Could you check a few things on this model? Use its own coordinates, in mm. Give positions to 0.01 mm unless a question says otherwise; leave off trailing zeros. Loops run counter-clockwise (first coordinate to the right, second up) from the corner with the lowest first, then second, coordinate; pieces in that order, holes last. Notation, with made-up numbers: M 47.5,35.25 L 61.5,35.25 A29 cw 61.5,65.25 Z; hole C -15.5,75 d10. An arc over 180 degrees is marked long. Return JSON: item names as keys, results as strings. Group by question number.
1. If we section it at C-C (y = 14.5): Write out the boundary of the cut face in (x, z), plus the area to 3 significant figures.
2. If we section it at A-A (x = 45.5): Write out the boundary of the cut face in (y, z).
3. Please list where these lines run through material, in increasing order: line 1 (Y direction, x = 45.5, z = 1.3); line 2 (Y direction, x = 45, z = 1.2); line 3 (X direction, y = 27.5, z = 0.7).
4. For pin 1 (2.5 mm diameter, centred on x = 14.5, y = 14.5, fed in from -Z); pin 2 (5 mm diameter, centred on x = 45.5, y = 14.5, fed in from -Z), each with a flat end and sliding along its axis, tell me the tip position at first contact or that it passes through.
5. If we section it at D-D (y = 26.5): Write out the boundary of the cut face in (x, z), plus the area to 3 significant figures.
6. If we section it at B-B (z = 1.4): Write out the boundary of the cut face in (x, y).
```python
from build123d import *

# Parameters (mm, degrees)
CROQUIS1_W              = 60
CROQUIS1_H              = 60
SALIENTE_EXTRUIR1_DEPTH = 2
CROQUIS7_R              = 1.6
CORTAR_EXTRUIR1_DEPTH   = 85.876380696
CROQUIS8_OUTSIDE_W      = 78.976
CROQUIS8_OUTSIDE_H      = 78.976
CORTAR_EXTRUIR2_DEPTH   = 10
CORTAR_EXTRUIR4_DEPTH   = 73.859453745
CHAFL_N1_SIZE           = 4


with BuildPart() as part:
    # Croquis1 → Saliente-Extruir1 (new body)
    with BuildSketch(Plane.XY):
        with Locations((30, 30)):
            Rectangle(CROQUIS1_W, CROQUIS1_H)
    extrude(amount=SALIENTE_EXTRUIR1_DEPTH)

    # Croquis7 → Cortar-Extruir1 (cut, through all)
    with BuildSketch(Plane.XY.offset(2)):
        with Locations((14.5, 45.5)):
            Circle(CROQUIS7_R)
        with Locations((45.5, 45.5)):
            Circle(CROQUIS7_R)
        with Locations((14.5, 14.5)):
            Circle(CROQUIS7_R)
        with Locations((45.5, 14.5)):
            Circle(CROQUIS7_R)
    extrude(amount=-CORTAR_EXTRUIR1_DEPTH, mode=Mode.SUBTRACT)

    # Croquis8 outside → Cortar-Extruir2 (cut)
    with BuildSketch(Plane(origin=(0, 0, 0), x_dir=(-1, 0, 0), z_dir=(0, 0, -1))):
        with Locations((-30, 30)):
            Rectangle(CROQUIS8_OUTSIDE_W, CROQUIS8_OUTSIDE_H)
        with BuildLine():
            Line((-51.5, 51.5), (-51.5, 8.5))
            Line((-51.5, 8.5), (-8.5, 8.5))
            Line((-8.5, 8.5), (-8.5, 36.95))
            ThreePointArc((-8.5, 36.95), (-16.379748932, 42.703353122), (-20.6, 51.5))
            Line((-20.6, 51.5), (-51.5, 51.5))
        make_face(mode=Mode.SUBTRACT)
    extrude(amount=-CORTAR_EXTRUIR2_DEPTH, mode=Mode.SUBTRACT)

    # Croquis10 → Cortar-Extruir4 (cut, through all)
    with BuildSketch(Plane(origin=(0, 0, 0), x_dir=(-1, 0, 0), z_dir=(0, 0, -1))):
        with BuildLine():
            ThreePointArc((-39.282790937, 18.384108052), (-37.770757205, 13.974782814), (-33.416887225, 12.30978694))
            ThreePointArc((-33.416887225, 12.30978694), (-23.815977303, 15.311202908), (-16.554661394, 22.2724715))
            ThreePointArc((-16.554661394, 22.2724715), (-17.629242795, 33.425217186), (-28.737692181, 34.888369193))
            ThreePointArc((-28.737692181, 34.888369193), (-35.948136426, 27.874421452), (-39.282790937, 18.384108052))
        make_face()
    extrude(amount=-CORTAR_EXTRUIR4_DEPTH, mode=Mode.SUBTRACT)

    # Chaflán1
    chafl_n1_edges = [part.edges().sort_by_distance(p)[0] for p in [
        (8.5, 8.5, 1),
        (51.5, 8.5, 1),
        (51.5, 51.5, 1),
    ]]
    chamfer(chafl_n1_edges, length=CHAFL_N1_SIZE)


solid = part.part
```
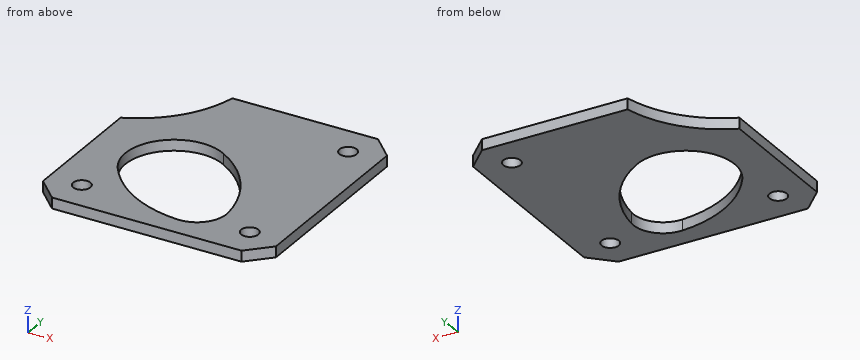
Answer:
{
 "1": {"outline": "M 8.5,0 L 12.9,0 L 12.9,2 L 8.5,2 Z; M 16.1,0 L 25.32,0 L 25.32,2 L 16.1,2 Z; M 38.22,0 L 43.9,0 L 43.9,2 L 38.22,2 Z; M 47.1,0 L 51.5,0 L 51.5,2 L 47.1,2 Z", "area": "47.4 mm²"},
 "2": {"outline": "M 8.5,0 L 12.9,0 L 12.9,2 L 8.5,2 Z; M 16.1,0 L 43.9,0 L 43.9,2 L 16.1,2 Z; M 47.1,0 L 51.5,0 L 51.5,2 L 47.1,2 Z"},
 "3": {"line 1": "y = 8.5 to 12.9, 16.1 to 43.9, 47.1 to 51.5", "line 2": "y = 8.5 to 12.98, 16.02 to 43.98, 47.02 to 51.5", "line 3": "x = 8.5 to 15.11, 36.18 to 51.5"},
 "4": {"pin 1": "passes through", "pin 2": "stops at z = 0"},
 "5": {"outline": "M 8.5,0 L 15.13,0 L 15.13,2 L 8.5,2 Z; M 36.76,0 L 51.5,0 L 51.5,2 L 36.76,2 Z", "area": "42.7 mm²"},
 "6": {"outline": "M 8.5,12.5 L 12.5,8.5 L 47.5,8.5 L 51.5,12.5 L 51.5,47.5 L 47.5,51.5 L 20.6,51.5 A20 cw 8.5,36.95 Z; hole C 14.5,14.5 d3.2; hole M 16.55,22.27 A22 ccw 33.42,12.31 A5.5 ccw 39.28,18.38 A22 ccw 28.74,34.89 A9 ccw Z; hole C 45.5,14.5 d3.2; hole C 45.5,45.5 d3.2"}
}
